```python
from build123d import *

# Parameters (mm, degrees)
ESQUISSE1_W             = 100
ESQUISSE1_H             = 100.548113933
ESQUISSE1_R             = 4
BOSS_EXTRU_1_DEPTH      = 8.5
ESQUISSE2_R             = 1.5
ENL_V_MAT_EXTRU_1_DEPTH = 73.637800077
ENL_V_MAT_EXTRU_6_DEPTH = 1
CONG_4_R                = 1
ESQUISSE4_R             = 3
ENL_V_MAT_EXTRU_7_DEPTH = 4


with BuildPart() as part:
    # Esquisse1 → Boss.-Extru.1 (new body)
    with BuildSketch(Plane.XY):
        with Locations((0, 1.725943033)):
            Rectangle(ESQUISSE1_W, ESQUISSE1_H)
        Circle(ESQUISSE1_R, mode=Mode.SUBTRACT)
    extrude(amount=BOSS_EXTRU_1_DEPTH)

    # Esquisse2 → Enlèv. mat.-Extru.1 (cut, through all)
    with BuildSketch(Plane.XY.offset(8.5)):
        with BuildLine():
            Line((27.5, 52), (27.5, 0))
            ThreePointArc((27.5, 0), (0, -27.5), (-27.5, 0))
            Line((-27.5, 0), (-27.5, 52))
            Line((-27.5, 52), (-50, 52))
            Line((-50, 52), (-50, -48.548113933))
            Line((-50, -48.548113933), (50, -48.548113933))
            Line((50, -48.548113933), (50, 52))
            Line((50, 52), (27.5, 52))
        make_face()
        with Locations((0, 22.5)):
            Circle(ESQUISSE2_R)
        with Locations((19.485571585, 11.25)):
            Circle(ESQUISSE2_R)
        with Locations((19.485571585, -11.25)):
            Circle(ESQUISSE2_R)
        with Locations((0, -22.5)):
            Circle(ESQUISSE2_R)
        with Locations((-19.485571585, -11.25)):
            Circle(ESQUISSE2_R)
        with Locations((-19.485571585, 11.25)):
            Circle(ESQUISSE2_R)
        with Locations((-15, 32)):
            Circle(ESQUISSE2_R)
        with Locations((15, 32)):
            Circle(ESQUISSE2_R)
    extrude(amount=-ENL_V_MAT_EXTRU_1_DEPTH, mode=Mode.SUBTRACT)

    # Esquisse3 → Enlèv. mat.-Extru.6 (cut)
    with BuildSketch(Plane.XY.offset(8.5)):
        with BuildLine():
            Line((27.5, 52), (-27.5, 52))
            Line((-27.5, 52), (-27.5, 20))
            Line((-27.5, 20), (-2.5, 20))
            Line((-2.5, 20), (-2.5, 22.5))
            ThreePointArc((-2.5, 22.5), (0, 25), (2.5, 22.5))
            Line((2.5, 22.5), (2.5, 20))
            Line((2.5, 20), (27.5, 20))
            Line((27.5, 20), (27.5, 52))
        make_face()
    extrude(amount=-ENL_V_MAT_EXTRU_6_DEPTH, mode=Mode.SUBTRACT)

    # Congé4
    cong_4_edges = [part.edges().sort_by_distance(p)[0] for p in [
        (-15, 20, 8.5),
        (15, 20, 8.5),
        (2.5, 21.25, 8.5),
        (-2.5, 21.25, 8.5),
        (0, 25, 8.5),
    ]]
    fillet(cong_4_edges, radius=CONG_4_R - 0.0001)  # a hair under: the kernel refuses the full size

    # Esquisse4 → Enlèv. mat.-Extru.7 (cut)
    with BuildSketch(Plane(origin=(0, 0, 0), x_dir=(-1, 0, 0), z_dir=(0, 0, -1))):
        with Locations((0, 22.5)):
            Circle(ESQUISSE4_R)
        with Locations((19.485571585, 11.25)):
            Circle(ESQUISSE4_R)
        with Locations((19.485571585, -11.25)):
            Circle(ESQUISSE4_R)
        with Locations((0, -22.5)):
            Circle(ESQUISSE4_R)
        with Locations((-19.485571585, -11.25)):
            Circle(ESQUISSE4_R)
        with Locations((-19.485571585, 11.25)):
            Circle(ESQUISSE4_R)
    extrude(amount=-ENL_V_MAT_EXTRU_7_DEPTH, mode=Mode.SUBTRACT)


solid = part.part
```
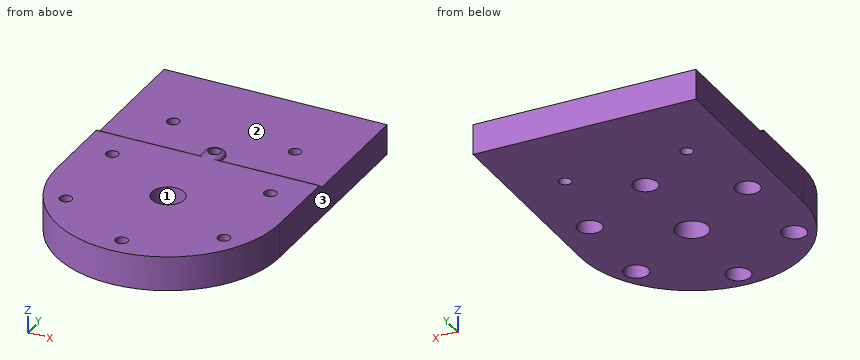
Input: part model. Units: mm. Frame: model coordinates. Face numbers are marked on the shaded views. Coordinates: 2 decimals unless noted, no trailing zeros. Write each loop counter-clockwise with the first axis right and the second up, starting at its lowest first coordinate (ties: lowest second). Pieces come first, ordered by that corner, then holes. Notation, with made-up numbers: (24.5, 86) - (30.5, 86) arc R35 cw to (30.5, 120) - close; hole circle Ø8 at (20, -19.75). An arc over 180 degrees is marked (long way). Put each result on its own line as item: value. Start each with the question number.
1) Mould query, pull axis X, two halves, no side actions, for the marked faces 1, 2 and 3. Classes: pulls with the +X half, pulls with the -X half, needs draft (parallel to the pull), parting line crosses it, or undercut.
2) Contact query for flat-ended pins moving along their axis: pin 1 (1 mm diameter, centred on x = -15.5, y = -16, fed in from -Z); pin 2 (5 mm diameter, centred on x = -19.49, y = 11.25, fed in from -Z); pin 3 (4 mm diameter, centred on x = 0, z = 5.5, fed in from -Y); pin 4 (1.5 mm diameter, centred on x = -11, z = 5.5, fed in from -Y). Output: stop coordinate, or through.
3) Cut plane C-C (y = -22.5). Return the cut outline in (x, z), plus the area to 3 significant figures.
4) Ray query, L1, parallel to Y at x = 0, z = 5.95; L2, parallel to Y at x = 0, z = 3.5; L3, parallel to Y at x = 17.5, z = 0.75. Return the intervals inside material, ascending.
5) Cut plane A-A (x = 0). State how many separate pieces and enclosed holes the cut face has, plus the area to 3 significant figures.
Resolved:
1. face 1: undercut
1. face 2: needs draft
1. face 3: pulls with the +X half
2. pin 1: stops at z = 0
2. pin 2: stops at z = 4
2. pin 3: stops at y = -27.5
2. pin 4: stops at y = -25.52
3. outline: (-15.81, 0) - (-3, 0) - (-3, 4) - (-1.5, 4) - (-1.5, 8.5) - (-15.81, 8.5) - close; (1.5, 4) - (3, 4) - (3, 0) - (15.81, 0) - (15.81, 8.5) - (1.5, 8.5) - close
3. area: 231 mm2
4. L1: y = -27.5 to -24, -21 to -4, 4 to 21, 24 to 52
4. L2: y = -27.5 to -25.5, -19.5 to -4, 4 to 19.5, 25.5 to 52
4. L3: y = -21.21 to -13.5, -9 to 9, 13.5 to 52
5. separate pieces: 4
5. enclosed holes: 0
5. area: 506 mm2
